from build123d import *

# Parameters (mm, degrees)
SKETCH1_R           = 44.45
BOSS_EXTRUDE1_DEPTH = 254
BOSS_EXTRUDE1_DRAFT = -4


# Read off the part's stored shape, not the designer's step: Revolve1
with BuildPart() as part:
    # Sketch1 → Boss-Extrude1 (with draft: the straight prism first)
    with BuildSketch(Plane.XY):
        Circle(SKETCH1_R)
    extrude(amount=-BOSS_EXTRUDE1_DEPTH)
    # Boss-Extrude1: the draft: its side faces are tilted about the plane it starts from
    boss_extrude1_sides = [part.faces().sort_by_distance(p)[0] for p in [
        (-44.45, 0, -127),
    ]]
    draft(boss_extrude1_sides, Plane.XY, BOSS_EXTRUDE1_DRAFT)

    # Revolve1 outline → Revolve1 (revolve)
    with BuildSketch(Plane.XZ):
        with BuildLine():
            Line((0, 0), (44.45, -4.4e-08))
            ThreePointArc((44.45, -4.4e-08), (31.430896439, 31.430896408), (0, 44.45))
            Line((0, 44.45), (0, 0))
        make_face()
    revolve(axis=Axis((0, 0, 0), (0, 0, 1)))

    # Sketch5 → Revolve2 (revolve)
    with BuildSketch(Plane(origin=(0, 0, 0), x_dir=(0, 0, -1), z_dir=(1, 0, 0))):
        with BuildLine():
            Line((254, 26.688589766), (254, -26.688589766))
            ThreePointArc((254, -26.688589766), (280.688589766, 0), (254, 26.688589766))
        make_face()
    revolve(axis=Axis((0, 26.688589766, -254), (0, -1, 0)))


solid = part.part
Here's how the part is built. I have some questions about the finished solid (model axes, mm). Coordinates: 2 decimals unless noted, no trailing zeros. Loops run counter-clockwise (first coordinate to the right, second up) from the corner with the lowest first, then second, coordinate; pieces in that order, holes last. Notation, with made-up numbers: (53.5, 11) -> (80.5, 11) arc R21 cw to (80.5, 50) -> close; hole circle Ø9 at (-34.5, 36). An arc over 180 degrees is marked (long way). Use one line per item in the form item = value. Start each with the question number.
(1) If we section it at A-A (x = 0): Please give me the cut outline in (y, z), then the cut area to 3 significant figures.
(2) If we section it at D-D (z = -25.5): Please give me the cut outline in (x, y), then the cut area to 3 significant figures.
(3) If we section it at C-C (z = -230.5): Please give me the cut outline in (x, y), then the cut area to 3 significant figures.
(4) Will these pins go through, and if not, where does the flat tip stop? pin 1 (6 mm diameter, centred on x = 18, z = -116, fed in from -Y); pin 2 (6 mm diameter, centred on y = -8, z = -146, fed in from -X); pin 3 (3 mm diameter, centred on x = 9.5, y = 30.5, fed in from +Z).
(5) Please list where these lines run through material, in increasing order: line 1 along X through (y, z) = (-15, -207); line 2 along Y through (x, z) = (-28, -72); line 3 along Y through (x, z) = (8, 31).
Verdict:
q1.outline = (-44.45, 0) -> (-26.69, -254) arc R26.69 ccw to (26.69, -254) -> (44.45, 0) arc R44.45 ccw to start
q1.area = 22,300 mm²
q2.outline = circle Ø85.33 at (0, 0)
q2.area = 5,720 mm²
q3.outline = circle Ø56.66 at (0, 0)
q3.area = 2,520 mm²
q4.pin_1 = -33.12
q4.pin_2 = -33.92
q4.pin_3 = 32.39
q5.line_1 = -25.95 to 25.95
q5.line_2 = -27.74 to 27.74
q5.line_3 = -30.84 to 30.84
